Read the model definition and answer for the solid it produces. Units are mm, in the model's axes. Give positions to 0.01 mm unless a question says otherwise; leave off trailing zeros. Loops run counter-clockwise (first coordinate to the right, second up) from the corner with the lowest first, then second, coordinate; pieces in that order, holes last. Notation, with made-up numbers: (53, 0) - (91, 0) arc R14 cw to (91, 24) - close; hole circle Ø7 at (56.5, 59). An arc over 180 degrees is marked (long way). Use a Markdown table: item, result. Add a question column.
Item 1: A cutting plane is placed at C-C (y = 1.45). Determine the outline of the cut face in (x, z), plus the area to 3 significant figures.
Item 2: A cutting plane is placed at B-B (x = 47). Determine the outline of the cut face in (y, z).
Item 3: A cutting plane is placed at D-D (z = 47.5). Determine the outline of the cut face in (x, y), plus the area to 3 significant figures.
Item 4: A cutting plane is placed at A-A (z = 2). Determine the outline of the cut face in (x, y), plus the area to 3 significant figures.
Item 5: Consider probe 1 along X at (y, z) = (0.55, 3); probe 2 along Z at (x, y) = (24, 0.7); probe 3 along X at (y, z) = (2.3, -20). Determine where each line is inside the solid, lowest interval first. Write a range as [from, to].
from build123d import *

# Parameters (mm, degrees)
Y_KSEKLIK_EKSTR_ZYON1_DEPTH = 3
KES_EKSTR_ZYON2_DEPTH       = 5.5


with BuildPart() as part:
    # Çizim1 → Yükseklik-Ekstrüzyon1 (new body)
    with BuildSketch(Plane(origin=(0, 0, 0), x_dir=(1, 0, 0), z_dir=(0, 1, 0))):
        with BuildLine():
            Line((-77.5, 24), (-77.5, -24))
            ThreePointArc((-77.5, -24), (0, -81.131066799), (77.5, -24))
            Line((77.5, -24), (77.5, 24))
            ThreePointArc((77.5, 24), (0, 81.131066799), (-77.5, 24))
        make_face()
    extrude(amount=Y_KSEKLIK_EKSTR_ZYON1_DEPTH)

    # Çizim4 → Kes-Ekstrüzyon2 (cut)
    with BuildSketch(Plane(origin=(0, 3, 0), x_dir=(1, 0, 0), z_dir=(0, 1, 0))):
        with BuildLine():
            Line((62.5, 20.404916559), (-0.5, 20.404916559))
            ThreePointArc((-0.5, 20.404916559), (-2.024235699, -1.095083441), (-0.5, -22.595083441))
            Line((-0.5, -22.595083441), (62.5, -22.595083441))
            ThreePointArc((62.5, -22.595083441), (64.017330872, -1.095083441), (62.5, 20.404916559))
        make_face()
    extrude(amount=-KES_EKSTR_ZYON2_DEPTH, mode=Mode.SUBTRACT)


solid = part.part
Geometry says:
| question | item | result |
|---|---|---|
| 1 | outline | (-77.5, -24) arc R81.13 ccw to (77.5, -24) - (77.5, 24) arc R81.13 ccw to (-77.5, 24) - close; hole (-0.5, -20.4) - (62.5, -20.4) arc R153.08 ccw to (62.5, 22.6) - (-0.5, 22.6) arc R152.4 ccw to start |
| 1 | area | 17,600 mm² |
| 2 | outline | (0, -66.13) - (3, -66.13) - (3, -20.4) - (0, -20.4) - close; (0, 22.6) - (3, 22.6) - (3, 66.13) - (0, 66.13) - close |
| 3 | outline | (-65.77, 0) - (65.77, 0) - (65.77, 3) - (-65.77, 3) - close |
| 3 | area | 395 mm² |
| 4 | outline | (-77.5, 0) - (-2.02, 0) - (-2.02, 3) - (-77.5, 3) - close; (64.01, 0) - (77.5, 0) - (77.5, 3) - (64.01, 3) - close |
| 4 | area | 267 mm² |
| 5 | probe 1 | [-77.5, -2.01], [64.01, 77.5] |
| 5 | probe 2 | [-77.5, -20.4], [22.6, 77.5] |
| 5 | probe 3 | [-77.5, -0.56], [62.56, 77.5] |
